```python
from build123d import *

# Parameters (mm, degrees)
F0_R     = 4
F1_DEPTH = 80
F2_W     = 72
F2_H     = 65
F3_DEPTH = 7.5581648407


with BuildPart() as f1:
    # F0 (on Top) → F1 (new body)
    with BuildSketch(Plane.XY):
        with BuildLine():
            Line((312.9912793082, 75.9082514048), (213.5049590409, 75.9082514048))
            ThreePointArc((213.5049590409, 75.9082514048), (211.7529694182, 75.5912560345), (210.2231288352, 74.6804643496))
            Line((210.2231288352, 74.6804643496), (149.8273279867, 22.1360384599))
            ThreePointArc((149.8273279867, 22.1360384599), (148.2974874037, 21.225246775), (146.545497781, 20.9082514048))
            Line((146.545497781, 20.9082514048), (-276.5839193761, 20.9082514048))
            ThreePointArc((-276.5839193761, 20.9082514048), (-280.1194532821, 19.4437853107), (-281.5839193761, 15.9082514048))
            Line((-281.5839193761, 15.9082514048), (-281.5839193761, -69.0917485952))
            ThreePointArc((-281.5839193761, -69.0917485952), (-280.1194532821, -72.6272825012), (-276.5839193761, -74.0917485952))
            Line((-276.5839193761, -74.0917485952), (312.9912793082, -74.0917485952))
            ThreePointArc((312.9912793082, -74.0917485952), (316.5268132142, -72.6272825012), (317.9912793082, -69.0917485952))
            Line((317.9912793082, -69.0917485952), (317.9912793082, 70.9082514048))
            ThreePointArc((317.9912793082, 70.9082514048), (316.5268132142, 74.4437853107), (312.9912793082, 75.9082514048))
        make_face()
        with Locations((-274.5839193761, -67.0917485952)):
            Circle(F0_R, mode=Mode.SUBTRACT)
        with Locations((310.9912793082, -67.0917485952)):
            Circle(F0_R, mode=Mode.SUBTRACT)
        with Locations((-274.5839193761, 13.9082514048)):
            Circle(F0_R, mode=Mode.SUBTRACT)
        with BuildLine():
            Line((-273.5839193761, -59.0917485952), (-273.5839193761, 5.9082514048))
            ThreePointArc((-273.5839193761, 5.9082514048), (-268.8711623353, 8.1954943639), (-266.5839193761, 12.9082514048))
            Line((-266.5839193761, 12.9082514048), (-112.4131828547, 12.9082514048))
            Line((-112.4131828547, 12.9082514048), (129.7935396433, 12.9082514048))
            ThreePointArc((129.7935396433, 12.9082514048), (139.4221907616, 4.3077632055), (149.5066444733, 12.3689735962))
            Line((149.5066444733, 12.3689735962), (215.8209085464, 69.4959036966))
            Line((215.8209085464, 69.4959036966), (221.9247751874, 69.4959036966))
            Line((221.9247751874, 69.4959036966), (302.9912793082, 69.4959036966))
            ThreePointArc((302.9912793082, 69.4959036966), (305.379178673, 63.1399404445), (311.7916584015, 60.9082514048))
            Line((311.7916584015, 60.9082514048), (311.7916584015, -59.0917485952))
            ThreePointArc((311.7916584015, -59.0917485952), (305.9541464058, -60.7847511051), (302.9912793082, -66.0917485952))
            Line((302.9912793082, -66.0917485952), (-266.5839193761, -66.0917485952))
            ThreePointArc((-266.5839193761, -66.0917485952), (-268.8711623353, -61.3789915544), (-273.5839193761, -59.0917485952))
        make_face(mode=Mode.SUBTRACT)
        with Locations((140.9914862647, 13.9082514048)):
            Circle(F0_R, mode=Mode.SUBTRACT)
        with Locations((310.9912793082, 68.9082514048)):
            Circle(F0_R, mode=Mode.SUBTRACT)
    extrude(amount=F1_DEPTH)

    # F2 (on face) → F3 (cut, through all)
    with BuildSketch(Plane(origin=(53.5865112104, -61.5935982634, 0), x_dir=(-0.754442589, -0.6563660411, 0), z_dir=(-0.6563660411, 0.754442589, 0))):
        with Locations((-166.607229352, 39.6668340825)):
            Rectangle(F2_W, F2_H)
    extrude(amount=-F3_DEPTH, mode=Mode.SUBTRACT)


solid = f1.part
```
The model under review builds one solid part; all positions refer to its coordinate system, in mm. A direction names the side the tool comes from. Round coordinates to 2 decimals unless told otherwise and drop trailing zeros. Write each loop counter-clockwise with the first axis right and the second up, starting at its lowest first coordinate (ties: lowest second). Pieces come first, ordered by that corner, then holes. Notation, with made-up numbers: (12, 84.5) -> (56, 84.5) arc R28 cw to (56, 108.5) -> close; hole circle Ø6 at (62.5, 25). An arc over 180 degrees is marked (long way). Use CSV: the item, a comma, the result in double quotes.
Q1. Consider section A-A (x = 84). Give the boundary of the cut face in (y, z).
Checks:
outline,"(-74.09, 0) -> (-66.09, 0) -> (-66.09, 80) -> (-74.09, 80) -> close; (12.91, 0) -> (20.91, 0) -> (20.91, 80) -> (12.91, 80) -> close"
Q2. Consider section C-C (z = 18). State how many separate pieces and enclosed holes the cut face has, then the cut area to 3 significant figures.
Checks:
separate pieces,"1"
enclosed holes,"5"
area,"10,500 mm²"
Q3. Mouldability with a two-part tool opening along Z and no side actions: class faces 4 (the flat face through (17, 18, 80)), 5 (the flat face through (182.2, 40.533, 74.996)), 6 (the flat face through (182, 45, 72.167)) as released by +Z, released by -Z, zero draft, split by the parting line, or undercut.
Checks:
face 4,"released by +Z"
face 5,"zero draft"
face 6,"undercut"
Q4. For pin 1 Ø9 at (x, y) = (140.99, 13.91) entering from -Z; pin 2 Ø24 at (x, z) = (-15.5, 50) entering from +Y, all flat-tipped, find the tip position at first contact; note any pin that passes through.
Checks:
pin 1,"z = 0"
pin 2,"y = 20.91"
Q5. For faces 1 (the flat face through (-281.584, -26, 39)), 2 (the flat face through (-62, 20.908, 39)), 3 (the flat face through (259, 69.496, 39)), list the 3-axis set-ups (+Z, -Z, +X, -X, +Y, -Y) from which the entire face can be reached by the end or side of a thin tool; tool diameter is ignored.
Checks:
face 1,"+Z, -Z, -X, +Y, -Y"
face 2,"+Z, -Z, -X, +Y"
face 3,"+Z, -Z"
Q6. Consider section B-B (y = -45.5). Give the boundary of the cut face in (x, z), then the cut area to 3 significant figures.
Checks:
outline,"(-281.58, 0) -> (-273.58, 0) -> (-273.58, 80) -> (-281.58, 80) -> close; (311.79, 0) -> (317.99, 0) -> (317.99, 80) -> (311.79, 80) -> close"
area,"1,140 mm²"
Q7. To check wall thickness, follow probe 1 along X at (y, z) = (3, 31.5); probe 2 along Y at (x, z) = (232, 61.5); probe 3 along Y at (x, z) = (-39, 38.5). State the ranges of each line that lie inside material, in increasing order. Write a range as [from, to].
Checks:
probe 1,"[-281.58, -273.58], [311.79, 317.99]"
probe 2,"[-74.09, -66.09], [69.5, 75.91]"
probe 3,"[-74.09, -66.09], [12.91, 20.91]"
